from build123d import *

# Parameters (mm, degrees)
F1_DEPTH = 100


with BuildPart() as f1:
    # F0 (on Top) → F1 (new body)
    with BuildSketch(Plane.XY):
        with BuildLine():
            Line((-5.698349, -4.52252), (-1.198349, -4.52252))
            Line((-1.198349, -4.52252), (1.301651, -4.52252))
            Line((1.301651, -4.52252), (4.569926, -7.790794))
            Line((4.569926, -7.790794), (4.569926, -8.52252))
            Line((4.569926, -8.52252), (0.801651, -8.52252))
            Line((0.801651, -8.52252), (0.801651, -9.52252))
            Line((0.801651, -9.52252), (1.301651, -9.52252))
            Line((1.301651, -9.52252), (1.301651, -10.02252))
            Line((1.301651, -10.02252), (3.365556, -10.02252))
            Line((3.365556, -10.02252), (6.301651, -10.02252))
            ThreePointArc((6.301651, -10.02252), (6.875677, -9.908339), (7.362312, -9.58318))
            Line((7.362312, -9.58318), (6.301651, -8.52252))
            Line((6.301651, -8.52252), (-0.253805, -1.967063))
            ThreePointArc((-0.253805, -1.967063), (-1.145969, -2.563188), (-2.198349, -2.77252))
            ThreePointArc((-2.198349, -2.77252), (-3.250728, -2.563188), (-4.142892, -1.967063))
            Line((-4.142892, -1.967063), (-10.698349, -8.52252))
            Line((-10.698349, -8.52252), (-11.759009, -9.58318))
            ThreePointArc((-11.759009, -9.58318), (-11.272374, -9.908339), (-10.698349, -10.02252))
            Line((-10.698349, -10.02252), (-7.762253, -10.02252))
            Line((-7.762253, -10.02252), (-5.698349, -10.02252))
            Line((-5.698349, -10.02252), (-5.698349, -9.52252))
            Line((-5.698349, -9.52252), (-5.198349, -9.52252))
            Line((-5.198349, -9.52252), (-5.198349, -8.52252))
            Line((-5.198349, -8.52252), (-8.966623, -8.52252))
            Line((-8.966623, -8.52252), (-8.966623, -7.790794))
            Line((-8.966623, -7.790794), (-5.698349, -4.52252))
        make_face()
        with BuildLine():
            ThreePointArc((-12.198349, -8.52252), (-12.084168, -9.096545), (-11.759009, -9.58318))
            Line((-11.759009, -9.58318), (-10.698349, -8.52252))
            Line((-10.698349, -8.52252), (-4.142892, -1.967063))
            ThreePointArc((-4.142892, -1.967063), (-4.739017, -1.074899), (-4.948349, -0.02252))
            ThreePointArc((-4.948349, -0.02252), (-4.739017, 1.02986), (-4.142892, 1.922024))
            Line((-4.142892, 1.922024), (-10.698349, 8.47748))
            Line((-10.698349, 8.47748), (-11.759009, 9.538141))
            ThreePointArc((-11.759009, 9.538141), (-12.084168, 9.051506), (-12.198349, 8.47748))
            Line((-12.198349, 8.47748), (-12.198349, 5.541385))
            Line((-12.198349, 5.541385), (-12.198349, 3.47748))
            Line((-12.198349, 3.47748), (-11.698349, 3.47748))
            Line((-11.698349, 3.47748), (-11.698349, 2.97748))
            Line((-11.698349, 2.97748), (-10.698349, 2.97748))
            Line((-10.698349, 2.97748), (-10.698349, 6.745755))
            Line((-10.698349, 6.745755), (-9.966623, 6.745755))
            Line((-9.966623, 6.745755), (-6.698349, 3.47748))
            Line((-6.698349, 3.47748), (-6.698349, -1.02252))
            Line((-6.698349, -1.02252), (-6.698349, -3.52252))
            Line((-6.698349, -3.52252), (-9.966623, -6.790794))
            Line((-9.966623, -6.790794), (-10.698349, -6.790794))
            Line((-10.698349, -6.790794), (-10.698349, -3.02252))
            Line((-10.698349, -3.02252), (-11.698349, -3.02252))
            Line((-11.698349, -3.02252), (-11.698349, -3.52252))
            Line((-11.698349, -3.52252), (-12.198349, -3.52252))
            Line((-12.198349, -3.52252), (-12.198349, -5.586424))
            Line((-12.198349, -5.586424), (-12.198349, -8.52252))
        make_face()
        with BuildLine():
            Line((-10.698349, 8.47748), (-4.142892, 1.922024))
            ThreePointArc((-4.142892, 1.922024), (-3.250728, 2.518149), (-2.198349, 2.72748))
            ThreePointArc((-2.198349, 2.72748), (-1.145969, 2.518149), (-0.253805, 1.922024))
            Line((-0.253805, 1.922024), (6.301651, 8.47748))
            Line((6.301651, 8.47748), (7.362312, 9.538141))
            ThreePointArc((7.362312, 9.538141), (6.875677, 9.8633), (6.301651, 9.97748))
            Line((6.301651, 9.97748), (3.365556, 9.97748))
            Line((3.365556, 9.97748), (1.301651, 9.97748))
            Line((1.301651, 9.97748), (1.301651, 9.47748))
            Line((1.301651, 9.47748), (0.801651, 9.47748))
            Line((0.801651, 9.47748), (0.801651, 8.47748))
            Line((0.801651, 8.47748), (4.569926, 8.47748))
            Line((4.569926, 8.47748), (4.569926, 7.745755))
            Line((4.569926, 7.745755), (1.301651, 4.47748))
            Line((1.301651, 4.47748), (-1.198349, 4.47748))
            Line((-1.198349, 4.47748), (-3.198349, 4.47748))
            Line((-3.198349, 4.47748), (-5.698349, 4.47748))
            Line((-5.698349, 4.47748), (-8.966623, 7.745755))
            Line((-8.966623, 7.745755), (-8.966623, 8.47748))
            Line((-8.966623, 8.47748), (-5.198349, 8.47748))
            Line((-5.198349, 8.47748), (-5.198349, 9.47748))
            Line((-5.198349, 9.47748), (-5.698349, 9.47748))
            Line((-5.698349, 9.47748), (-5.698349, 9.97748))
            Line((-5.698349, 9.97748), (-7.762253, 9.97748))
            Line((-7.762253, 9.97748), (-10.698349, 9.97748))
            ThreePointArc((-10.698349, 9.97748), (-11.272374, 9.8633), (-11.759009, 9.538141))
            Line((-11.759009, 9.538141), (-10.698349, 8.47748))
        make_face()
        with BuildLine():
            Line((6.301651, -8.52252), (7.362312, -9.58318))
            ThreePointArc((7.362312, -9.58318), (7.687471, -9.096545), (7.801651, -8.52252))
            Line((7.801651, -8.52252), (7.801651, -5.586424))
            Line((7.801651, -5.586424), (7.801651, -3.52252))
            Line((7.801651, -3.52252), (7.301651, -3.52252))
            Line((7.301651, -3.52252), (7.301651, -3.02252))
            Line((7.301651, -3.02252), (6.301651, -3.02252))
            Line((6.301651, -3.02252), (6.301651, -6.790794))
            Line((6.301651, -6.790794), (5.569926, -6.790794))
            Line((5.569926, -6.790794), (2.301651, -3.52252))
            Line((2.301651, -3.52252), (2.301651, -1.02252))
            Line((2.301651, -1.02252), (2.301651, 0.97748))
            Line((2.301651, 0.97748), (2.301651, 3.47748))
            Line((2.301651, 3.47748), (5.569926, 6.745755))
            Line((5.569926, 6.745755), (6.301651, 6.745755))
            Line((6.301651, 6.745755), (6.301651, 2.97748))
            Line((6.301651, 2.97748), (7.301651, 2.97748))
            Line((7.301651, 2.97748), (7.301651, 3.47748))
            Line((7.301651, 3.47748), (7.801651, 3.47748))
            Line((7.801651, 3.47748), (7.801651, 5.541385))
            Line((7.801651, 5.541385), (7.801651, 8.47748))
            ThreePointArc((7.801651, 8.47748), (7.687471, 9.051506), (7.362312, 9.538141))
            Line((7.362312, 9.538141), (6.301651, 8.47748))
            Line((6.301651, 8.47748), (-0.253805, 1.922024))
            ThreePointArc((-0.253805, 1.922024), (0.34232, 1.02986), (0.551651, -0.02252))
            ThreePointArc((0.551651, -0.02252), (0.34232, -1.074899), (-0.253805, -1.967063))
            Line((-0.253805, -1.967063), (6.301651, -8.52252))
        make_face()
    extrude(amount=F1_DEPTH)


solid = f1.part
Verification items for the finished model (mm, model axes). A direction names the side the tool comes from. Give positions to 0.01 mm unless a question says otherwise; leave off trailing zeros.
1. Go/stop test with flat-tipped pins: P1, Ø2, axis at x = -4.5, z = 16, coming from the +Y side; P2, Ø0.5, axis at y = 9, z = 26, coming from the -X side; P3, Ø0.6, axis at x = -12, z = 74, coming from the +Y side. Record where each tip stops, or that it passes through.
Derived:
P1: stops at y = 9.48
P2: stops at x = -12.17
P3: stops at y = 9.59
2. Release check for a two-part mould opening along Y. For faces 1 (the flat face through (4, -10.023, 49)), 2 (the flat face through (-7, 8.477, 49)), 3 (the flat face through (-8.31, -5.134, 49.3)), 4 (the flat face through (0, -2, 0)) record: +Y half, -Y half, draft (parallel to the pull), parting line (faces both ways), or undercut.
Derived:
face 1: -Y half
face 2: undercut
face 3: undercut
face 4: draft
3. Tool access check on faces 5 (the flat face through (2.91, -6.13, 49.3)), 6 (the flat face through (7.802, 6, 49)). Record the directions out of +Z, -Z, +X, -X, +Y, -Y that give a thin tool (end or side, any length) a straight path to the whole face; none if there is none.
Derived:
face 5: +Z, -Z
face 6: +Z, -Z, +X, +Y, -Y
4. Material ranges on probe 1 along Y at (x, z) = (-10.25, 10); probe 2 along X at (y, z) = (-8, 25); probe 3 along Y at (x, z) = (-6.75, 82), recorded low to high.
Derived:
probe 1: y = -10.02 to -6.79, 6.75 to 9.98
probe 2: x = -12.2 to -8.97, 4.57 to 7.8
probe 3: y = -10.02 to -8.52, -5.57 to -3.57, 3.53 to 5.53, 8.48 to 9.98
